Read the model definition and answer for the solid it produces. Units are mm, in the model's axes. Face numbers are marked on the shaded views. A direction names the side the tool comes from. Round coordinates to 2 decimals unless told otherwise and drop trailing zeros. Write each loop counter-clockwise with the first axis right and the second up, starting at its lowest first coordinate (ties: lowest second). Pieces come first, ordered by that corner, then holes. Notation, with made-up numbers: (17.5, -15) -> (72.5, -15) arc R27 cw to (72.5, 7) -> close; hole circle Ø5 at (-21, 29). An arc over 180 degrees is marked (long way). Return JSON: item names as keys, results as strings.
from build123d import *

# Parameters (mm, degrees)
F0_R     = 10
F1_DEPTH = 10
F2_R     = 7.5
F3_DEPTH = 10
F5_R     = 17
F6_DEPTH = 3
F7_R     = 10
F8_DEPTH = 50.501


with BuildPart() as f1:
    # F0 (on Top) → F1 (new body)
    with BuildSketch(Plane.XY):
        with BuildLine():
            Line((-30, -15), (-13.228757, -15))
            ThreePointArc((-13.228757, -15), (0, -20), (13.228757, -15))
            Line((13.228757, -15), (30, -15))
            Line((30, -15), (30, 15))
            Line((30, 15), (13.228757, 15))
            ThreePointArc((13.228757, 15), (0, 20), (-13.228757, 15))
            Line((-13.228757, 15), (-30, 15))
            Line((-30, 15), (-30, -15))
        make_face()
        Circle(F0_R, mode=Mode.SUBTRACT)
    extrude(amount=F1_DEPTH)

    # F2 (on face) → F3 (join)
    with BuildSketch(Plane.YZ.offset(30)):
        with BuildLine():
            Line((-15, 32.5), (-15, 10))
            Line((-15, 10), (15, 10))
            Line((15, 10), (15, 32.5))
            ThreePointArc((15, 32.5), (0, 47.5), (-15, 32.5))
        make_face()
        with Locations((0, 32.5)):
            Circle(F2_R, mode=Mode.SUBTRACT)
    extrude(amount=-F3_DEPTH)

    # F4: F1 across plane


with BuildPart() as f1_1:
    add(f1.part)
    add(f1.part.mirror(Plane.YZ))

    # F5 (on face) → F6 (join)
    with BuildSketch(Plane(origin=(0, 0, 0), x_dir=(1, 0, 0), z_dir=(0, 0, -1))):
        Circle(F5_R)
    extrude(amount=F6_DEPTH)

    # F7 (on face) → F8 (cut, through all)
    with BuildSketch(Plane(origin=(0, 0, -3), x_dir=(1, 0, 0), z_dir=(0, 0, -1))):
        Circle(F7_R)
    extrude(amount=-F8_DEPTH, mode=Mode.SUBTRACT)


solid = f1_1.part
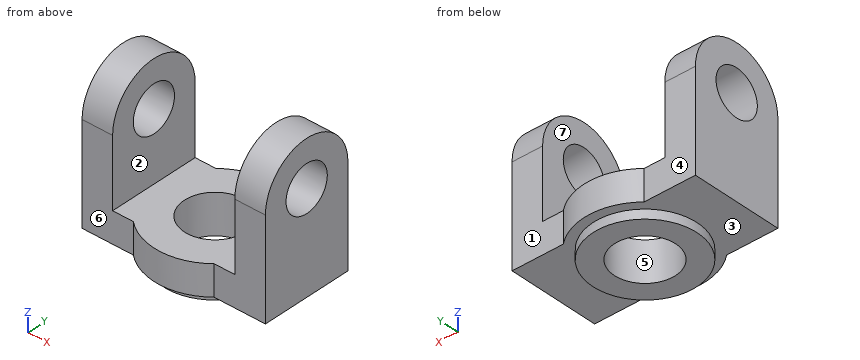
Item 1: Section C-C (z = 14) is taken. Give the vertices of the cut face in (x, y).
Worked answers:
{"outline": "(-30, -15) -> (-20, -15) -> (-20, 15) -> (-30, 15) -> close; (20, -15) -> (30, -15) -> (30, 15) -> (20, 15) -> close"}
Item 2: For a pull along Y with two mould halves and no side action, classify the marked faces 5, 6 and 7 as released by +Y, released by -Y, zero draft, split by the parting line, or undercut.
Worked answers:
{"face 5": "undercut", "face 6": "released by -Y", "face 7": "zero draft"}
Item 3: Section D-D (z = 30) is taken. Give the vertices of the cut face in (x, y), then the cut area to 3 significant figures.
Worked answers:
{"outline": "(-30, -15) -> (-20, -15) -> (-20, -7.07) -> (-30, -7.07) -> close; (-30, 7.07) -> (-20, 7.07) -> (-20, 15) -> (-30, 15) -> close; (20, -15) -> (30, -15) -> (30, -7.07) -> (20, -7.07) -> close; (20, 7.07) -> (30, 7.07) -> (30, 15) -> (20, 15) -> close", "area": "317 mm2"}
Item 4: Section B-B (x = -26) is taken. Give the vertices of the cut face in (y, z).
Worked answers:
{"outline": "(-15, 0) -> (15, 0) -> (15, 32.5) arc R15 ccw to (-15, 32.5) -> close; hole circle Ø15 at (0, 32.5)"}
Item 5: A tool of negligible diameter and unlimited length cuts with its end or side. For the marked faces 1, 2, 3 and 4, from which of +Z, -Z, +X, -X, +Y, -Y can it reach the whole face along a straight path? Write none if from no direction.
Worked answers:
{"face 1": "+Z, -Z, +X, +Y", "face 2": "+Z, +Y, -Y", "face 3": "-Z", "face 4": "+Z, -Z, -X, +Y"}
Item 6: Section A-A (y = 0) is taken. Give the vertices of the cut face in (x, z).
Worked answers:
{"outline": "(-30, 0) -> (-17, 0) -> (-17, -3) -> (-10, -3) -> (-10, 10) -> (-20, 10) -> (-20, 25) -> (-30, 25) -> close; (-30, 40) -> (-20, 40) -> (-20, 47.5) -> (-30, 47.5) -> close; (10, -3) -> (17, -3) -> (17, 0) -> (30, 0) -> (30, 25) -> (20, 25) -> (20, 10) -> (10, 10) -> close; (20, 40) -> (30, 40) -> (30, 47.5) -> (20, 47.5) -> close"}
Item 7: Flat-ended cylindrical pins translate along their axes: pin 1 (13.5 mm diameter, centred on x = -22, z = 16.5, fed in from +Y); pin 2 (24 mm diameter, centred on y = 0, z = 32.5, fed in from +X); pin 3 (5 mm diameter, centred on x = 18, z = 9.5, fed in from -Y); pin 4 (20 mm diameter, centred on x = 4, y = -3.5, fed in from +Z). Find the tip coordinate at first contact, or state that the pin passes through.
Worked answers:
{"pin 1": "stops at y = 15", "pin 2": "stops at x = 30", "pin 3": "stops at y = -15", "pin 4": "stops at z = 10"}
Item 8: Straight lines are drawn through the part: L1, parallel to X at y = -2.5, z = 21; L2, parallel to Z at x = -27.5, y = 0; L3, parallel to Y at x = 0, z = 5. For each, find the intervals that lie inside material, in ascending order. Write a range as [from, to].
Worked answers:
{"L1": "x = [-30, -20], [20, 30]", "L2": "z = [0, 25], [40, 47.5]", "L3": "y = [-20, -10], [10, 20]"}
